For this review, take the finished solid that the model builds, in its own axes (mm). Face numbers are marked on the shaded views. A direction names the side the tool comes from. Coordinates: 2 decimals unless noted, no trailing zeros. Write each loop counter-clockwise with the first axis right and the second up, starting at its lowest first coordinate (ties: lowest second). Pieces come first, ordered by that corner, then holes.
```python
from build123d import *

# Parameters (mm, degrees)
SKETCH_W        = 85.5
SKETCH_H        = 20
PAD_DEPTH       = 127.2
PAD_FACE5_W     = 20
PAD_FACE5_H     = 85.5
POCKET_DEPTH    = 1.88
POCKET001_DEPTH = 20.001


with BuildPart() as part:
    # Sketch → Pad (new body)
    with BuildSketch(Plane.XY):
        Rectangle(SKETCH_W, SKETCH_H)
    extrude(amount=PAD_DEPTH)

    # Pad Face5 → Pocket (cut)
    with BuildSketch(Plane(origin=(0, 0, 0), x_dir=(0, -1, 0), z_dir=(0, 0, -1))):
        Rectangle(PAD_FACE5_W, PAD_FACE5_H)
    extrude(amount=-POCKET_DEPTH, mode=Mode.SUBTRACT)

    # Sketch001 (on Face1 of Pocket) → Pocket001 (cut, through all)
    with BuildSketch(Plane.XZ.offset(10)):
        Polygon((13.325244, 70.04), (26.650488, 93.12), (13.325244, 116.2), (-13.325244, 116.2), (-26.650488, 93.12), (-13.325244, 70.04), align=None)
        Polygon((13.325244, 12.88), (26.650488, 35.96), (13.325244, 59.04), (-13.325244, 59.04), (-26.650488, 35.96), (-13.325244, 12.88), align=None)
    extrude(amount=-POCKET001_DEPTH, mode=Mode.SUBTRACT)


solid = part.part
```
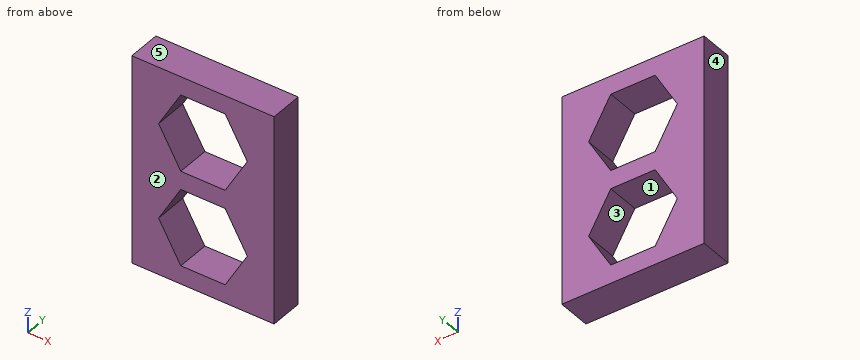
Q1. Add section D-D (z = 16). State the section outline as (x, y) points, then the cut area to 3 significant figures.
Ans:
outline: (-42.75, -10) - (-15.13, -10) - (-15.13, 10) - (-42.75, 10) - close; (15.13, -10) - (42.75, -10) - (42.75, 10) - (15.13, 10) - close
area: 1,100 mm2
Q2. Draft analysis for pull direction X (two halves, no side actions). For the marked faces 3, 4 and 5, state which applies: +X half, -X half, draft (parallel to the pull), parting line (faces both ways), or undercut.
Ans:
face 3: undercut
face 4: -X half
face 5: draft
Q3. Add section A-A (x = 7.5). State the section outline as (y, z) points, then the cut area to 3 significant figures.
Ans:
outline: (-10, 1.88) - (10, 1.88) - (10, 12.88) - (-10, 12.88) - close; (-10, 59.04) - (10, 59.04) - (10, 70.04) - (-10, 70.04) - close; (-10, 116.2) - (10, 116.2) - (10, 127.2) - (-10, 127.2) - close
area: 660 mm2
Q4. Add section C-C (y = -7). State the section outline as (x, z) points.
Ans:
outline: (-42.75, 1.88) - (42.75, 1.88) - (42.75, 127.2) - (-42.75, 127.2) - close; hole (-26.65, 35.96) - (-13.33, 12.88) - (13.33, 12.88) - (26.65, 35.96) - (13.33, 59.04) - (-13.33, 59.04) - close; hole (-26.65, 93.12) - (-13.33, 70.04) - (13.33, 70.04) - (26.65, 93.12) - (13.33, 116.2) - (-13.33, 116.2) - close
Q5. Tool access review of the marked faces 1 and 2: name each direction out of +Z, -Z, +X, -X, +Y, -Y from which nothing blocks a thin tool from reaching the whole face with its end or side.
Ans:
face 1: +Y, -Y
face 2: +Z, -Z, +X, -X, -Y
Q6. Add section B-B (z = 34.5). State the section outline as (x, y) points, then the cut area to 3 significant figures.
Ans:
outline: (-42.75, -10) - (-25.81, -10) - (-25.81, 10) - (-42.75, 10) - close; (25.81, -10) - (42.75, -10) - (42.75, 10) - (25.81, 10) - close
area: 678 mm2
Q7. For probe 1 along Z at (x, y) = (-6, 3.5); probe 2 along Z at (x, y) = (-22, 0.5); probe 3 along X at (y, z) = (-5, 22), list the stretches that pass through material, from the lowest coordinate up.
Ans:
probe 1: z = 1.88 to 12.88, 59.04 to 70.04, 116.2 to 127.2
probe 2: z = 1.88 to 27.91, 44.01 to 85.07, 101.17 to 127.2
probe 3: x = -42.75 to -18.59, 18.59 to 42.75
